from build123d import *

# Parameters (mm, degrees)
BOSS_EXTRUDE1_DEPTH     = 60.96
CUT_EXTRUDE1_DEPTH      = 3.81
CUT_EXTRUDE1_DEPTH_BACK = 3.81
SKETCH4_W               = 44.196
SKETCH4_H               = 36.576
SKETCH6_R               = 12.065
SKETCH6_R_2             = 3.81
CUT_EXTRUDE2_DEPTH      = 40.64
CUT_EXTRUDE4_DEPTH      = 126.82636128
CUT_EXTRUDE4_DEPTH_BACK = 126.82636128
FILLET1_R               = 3.556


with BuildPart() as part:
    # Sketch2 → Boss-Extrude1 (new body)
    with BuildSketch(Plane.XY):
        with BuildLine():
            Line((-35.382985005, -21.149184515), (-35.382985005, 15.680815485))
            ThreePointArc((-35.382985005, 15.680815485), (-33.145202484, 26.105386529), (-26.826159694, 34.693113252))
            ThreePointArc((-26.826159694, 34.693113252), (-24.077840328, 38.155820727), (-22.682985005, 42.350815485))
            Line((-22.682985005, 42.350815485), (3.352014995, 42.350815485))
            Line((3.352014995, 42.350815485), (3.352014995, 38.540815485))
            Line((3.352014995, 38.540815485), (27.482014995, 38.540815485))
            Line((27.482014995, 38.540815485), (27.482014995, 42.350815485))
            Line((27.482014995, 42.350815485), (53.517014995, 42.350815485))
            ThreePointArc((53.517014995, 42.350815485), (54.911870318, 38.155820727), (57.660189685, 34.693113252))
            ThreePointArc((57.660189685, 34.693113252), (63.979232475, 26.105386529), (66.217014995, 15.680815485))
            Line((66.217014995, 15.680815485), (66.217014995, -21.149184515))
            Line((66.217014995, -21.149184515), (56.057014995, -21.149184515))
            Line((56.057014995, -21.149184515), (56.057014995, 9.330815485))
            ThreePointArc((56.057014995, 9.330815485), (52.337271116, 18.311071606), (43.357014995, 22.030815485))
            Line((43.357014995, 22.030815485), (-12.522985005, 22.030815485))
            ThreePointArc((-12.522985005, 22.030815485), (-21.503241126, 18.311071606), (-25.222985005, 9.330815485))
            Line((-25.222985005, 9.330815485), (-25.222985005, -21.149184515))
            Line((-25.222985005, -21.149184515), (-35.382985005, -21.149184515))
        make_face()
    extrude(amount=-BOSS_EXTRUDE1_DEPTH)

    # Sketch4 → Cut-Extrude1 (cut, two sides: drawn at the far end of the back side and taken through both)
    with BuildSketch(Plane(origin=(0, 38.540815485, 0), x_dir=(1, 0, 0), z_dir=(0, 1, 0)).offset(-CUT_EXTRUDE1_DEPTH_BACK)):
        with Locations((15.417014995, 30.48)):
            Rectangle(SKETCH4_W, SKETCH4_H)
    extrude(amount=CUT_EXTRUDE1_DEPTH + CUT_EXTRUDE1_DEPTH_BACK, mode=Mode.SUBTRACT)

    # Sketch6 → Cut-Extrude2 (cut)
    with BuildSketch(Plane(origin=(0, 42.350815485, 0), x_dir=(1, 0, 0), z_dir=(0, 1, 0))):
        with Locations(Location((15.417014995, 30.48, 0), (0, 0, 270))):
            Circle(SKETCH6_R)
        with Locations(Location((-15.062985005, 8.255, 0), (0, 0, 270))):
            Circle(SKETCH6_R_2)
        with Locations(Location((-15.062985005, 52.705, 0), (0, 0, 270))):
            Circle(SKETCH6_R_2)
        with Locations(Location((45.897014995, 52.705, 0), (0, 0, 270))):
            Circle(SKETCH6_R_2)
        with Locations(Location((45.897014995, 8.255, 0), (0, 0, 270))):
            Circle(SKETCH6_R_2)
    extrude(amount=-CUT_EXTRUDE2_DEPTH, mode=Mode.SUBTRACT)

    # Sketch7 → Cut-Extrude4 (cut, two sides: drawn at the far end of the back side and taken through both)
    with BuildSketch(Plane(origin=(66.217014995, 0, 0), x_dir=(0, 0, -1), z_dir=(1, 0, 0)).offset(-CUT_EXTRUDE4_DEPTH_BACK)):
        with BuildLine():
            Line((12.7, -1.591184515), (12.7, -21.149184515))
            Line((12.7, -21.149184515), (48.26, -21.149184515))
            Line((48.26, -21.149184515), (48.26, -1.591184515))
            ThreePointArc((48.26, -1.591184515), (30.48, 10.61965618), (12.7, -1.591184515))
        make_face()
    extrude(amount=CUT_EXTRUDE4_DEPTH + CUT_EXTRUDE4_DEPTH_BACK, mode=Mode.SUBTRACT)

    # Fillet1
    fillet1_edges = [part.edges().sort_by_distance(p)[0] for p in [
        (37.515014995, 38.540815485, -12.192),
        (37.515014995, 38.540815485, -48.768),
        (-6.680985005, 38.540815485, -48.768),
        (-6.680985005, 38.540815485, -12.192),
    ]]
    fillet(fillet1_edges, radius=FILLET1_R)


solid = part.part
Design review of the part built by this model. Coordinates are the model's own, in mm. A direction names the side the tool comes from. Round coordinates to 2 decimals unless told otherwise and drop trailing zeros. Order: outer loops, then holes, each group sorted by start corner. A loop starts at its lowest first (then second) coordinate and runs counter-clockwise, first axis right, second up.
1) Draft analysis for pull direction Z (two halves, no side actions). For faces 1 (the flat face through (27.482, 40, -55)), 2 (the flat face through (15, 38, -12.192)), state which applies: released by +Z, released by -Z, zero draft, split by the parting line, or undercut.
The answers:
face 1: zero draft
face 2: undercut
2) Consider section A-A (z = -30.48). State the section outline as (x, y) points.
The answers:
outline: (-35.38, 10.62) - (-25.16, 10.62) arc R12.7 cw to (-12.52, 22.03) - (3.35, 22.03) - (3.35, 34.73) - (-6.68, 34.73) - (-6.68, 42.35) - (-22.68, 42.35) arc R12.7 cw to (-26.83, 34.69) arc R25.4 ccw to (-35.38, 15.68) - close; (27.48, 22.03) - (43.36, 22.03) arc R12.7 cw to (55.99, 10.62) - (66.22, 10.62) - (66.22, 15.68) arc R25.4 ccw to (57.66, 34.69) arc R12.7 cw to (53.52, 42.35) - (37.52, 42.35) - (37.52, 34.73) - (27.48, 34.73) - close
3) Clearance check with flat-ended pins moving along their axes: pin 1 Ø1 at (x, z) = (38.5, -19) entering from -Y; pin 2 Ø6 at (x, y) = (6.5, 39.5) entering from +Z; pin 3 Ø3.5 at (x, z) = (12, -3) entering from +Y; pin 4 Ø4 at (y, z) = (33, -44.5) entering from -X. State where each tip first meets the part, or that it passes through.
The answers:
pin 1: stops at y = 22.03
pin 2: stops at z = 0
pin 3: stops at y = 38.54
pin 4: stops at x = -30.24
4) Consider section B-B (y = -3). State the section outline as (x, z) points.
The answers:
outline: (-35.38, -60.96) - (-25.22, -60.96) - (-25.22, -48.26) - (-35.38, -48.26) - close; (-35.38, -12.7) - (-25.22, -12.7) - (-25.22, 0) - (-35.38, 0) - close; (56.06, -60.96) - (66.22, -60.96) - (66.22, -48.26) - (56.06, -48.26) - close; (56.06, -12.7) - (66.22, -12.7) - (66.22, 0) - (56.06, 0) - close
5) Consider section D-D (x = 22.5). State the section outline as (y, z) points.
The answers:
outline: (22.03, -60.96) - (38.54, -60.96) - (38.54, -48.77) - (34.73, -48.77) - (34.73, -40.25) - (22.03, -40.25) - close; (22.03, -20.71) - (34.73, -20.71) - (34.73, -12.19) - (38.54, -12.19) - (38.54, 0) - (22.03, 0) - close
6) For L1, parallel to X at y = 8, z = -8; L2, parallel to Z at x = -12, y = 33; L3, parallel to X at y = 28, z = -52, list the stretches that pass through material, from the lowest coordinate up.
The answers:
L1: x = -35.38 to -25.22, 56.06 to 66.22
L2: z = -60.96 to -54.97, -50.44 to -10.52, -5.99 to 0
L3: x = -32.2 to -18.81, -11.32 to 42.15, 49.64 to 63.03
7) Machinability: for faces 3 (the flat face through (61, -21.149, -55)), 4 (the flat face through (56.057, -6, -54)), 5 (the cylindrical face through (-5.667, 38.594, -47.699)), 6 (the flat face through (61, -11, -12.7)), which of the approach directions +Z, -Z, +X, -X, +Y, -Y give a long, thin tool a straight path to every point of the face, cutting with its end or side? Answer none if there is none.
The answers:
face 3: +Z, -Z, +X, -X, -Y
face 4: +Z, -Z, -Y
face 5: +Y
face 6: +X, -X, -Y
8) Consider section C-C (y = 18). State the section outline as (x, z) points.
The answers:
outline: (-35.28, -60.96) - (-21.8, -60.96) - (-21.8, 0) - (-35.28, 0) - close; (52.64, -60.96) - (66.11, -60.96) - (66.11, 0) - (52.64, 0) - close
